Part model, mm, in its own coordinate system. A direction names the side the tool comes from. Round coordinates to 2 decimals unless told otherwise and drop trailing zeros. Loops run counter-clockwise (first coordinate to the right, second up) from the corner with the lowest first, then second, coordinate; pieces in that order, holes last. Notation, with made-up numbers: M 43.5,87 L 70.5,87 A13 ccw 70.5,104 Z; hole C 78,12 d11. An arc over 180 degrees is marked long. Put each result on its own line as item: value. Start each with the question number.
1) Probe line 1 along Y through (x, z) = (4.25, -0.5); line 2 along Y through (x, z) = (-4, -2); line 3 along X through (y, z) = (58, -0.25). List the from-to ranges inside material, lowest first.
2) Pull direction X, two halves, no side cores. Call faces 1 (the cylindrical face through (0.69, 37.57, 3.1)), 2 (the flat face through (-2.05, 80.98, 1.21)), 3 (the flat face through (0, 0, 0)): +X half, -X half, draft (parallel to the pull), parting line (faces both ways), or undercut.
3) Slice it at B-B on y = 57. Give the cut face in (x, z) (3 decimals), then the cut area to 3 significant figures.
4) Which spindle directions (+Z, -Z, +X, -X, +Y, -Y) get a long thin tool onto all of the face, cutting with end or side? Do faces 4 (the flat face through (1, 76.2, -4)), 5 (the flat face through (2, 82.55, 2)), 6 (the flat face through (0, 81, 2.381)). Say none if no direction does.
5) Drop flat-ended pins along their axis: pin 1 Ø1 at (x, z) = (-0.5, 1.5) entering from +Y (3 decimals); pin 2 Ø3 at (y, z) = (50.5, -1) entering from +X (3 decimals); pin 3 Ø2 at (x, y) = (-1.5, 8.5) entering from -Z. Give the stop position or say it passes through.
Autodesk Inventor part; units mm, degrees
ref_plane "YZ Plane" through (0, 0, 0) normal (1, 0, 0) x (0, 1, 0)
ref_plane "XZ Plane" through (0, 0, 0) normal (0, 1, 0) x (-1, 0, 0)
ref_plane "XY Plane" through (0, 0, 0) normal (0, 0, 1) x (1, 0, 0)
sketch "Sketch1" plane through (0, 0, 0) normal (0, 1, 0) x (-1, 0, 0)
  circle A0 centre (0, 0) radius 3.175
  dimension "d0" = 6.35
extrude "Extrusion1" add sketch "Sketch1" along normal blind 76.2
sketch "Sketch2" plane through (0, 76.2, 0) normal (0, 1, 0) x (1, 0, 0)
  circle A0 centre (0, 0) radius 3.175
  circle A1 centre (0, 0) radius 4.7625
  dimension "d3" = 9.525
extrude "Extrusion2" add sketch "Sketch2" along normal blind 6.35 contours A0 | A1
sketch "Sketch3" plane through (0, 82.55, 0) normal (0, 1, 0) x (1, 0, 0)
  circle A0 centre (0, 0) radius 4.7625
  line L0 (-1.3748, 2.3812) -> (1.3748, 2.3813)
  line L1 (1.3748, 2.3813) -> (2.7496, 0)
  line L2 (2.7496, 0) -> (1.3748, -2.3813)
  line L3 (1.3748, -2.3813) -> (-1.3748, -2.3813)
  line L4 (-1.3748, -2.3813) -> (-2.7496, 0)
  line L5 (-2.7496, 0) -> (-1.3748, 2.3812)
  dimension "d6" = 4.7625
extrude "Extrusion3" cut sketch "Sketch3" against normal blind 3.175 contours L0 L1 L2 L3 L4 L5
fillet "Fillet1" radius 0.3969 3 edges at (3.175, 76.2, 0) (-4.7625, 82.55, 0) (3.175, 0, 0)
properties part number "Bolt_0.25_20_3.0len_SocketHead" material "Stainless Steel, Austenitic"
Recorded:
1. line 1: y = 76.2 to 82.55
1. line 2: y = 76.2 to 82.54
1. line 3: x = -3.17 to 3.17
2. face 1: parting line
2. face 2: undercut
2. face 3: draft
3. outline: C 0,0 d6.35
3. area: 31.7 mm2
4. face 4: -Y
4. face 5: +Z, -Z, +X, -X, +Y
4. face 6: +Y
5. pin 1: stops at y = 79.375
5. pin 2: stops at x = 3.175
5. pin 3: stops at z = -3.14
